Here's how the part is built. I have some questions about the finished solid (model axes, mm). A direction names the side the tool comes from. Round coordinates to 2 decimals unless told otherwise and drop trailing zeros. Order: outer loops, then holes, each group sorted by start corner. A loop starts at its lowest first (then second) coordinate and runs counter-clockwise, first axis right, second up. Notation, with made-up numbers: (-20, -25.5) - (-5, -25.5) arc R37 cw to (-5, 12.5) - close; hole circle Ø4 at (87, -37). An arc over 180 degrees is marked (long way). Answer as a JSON object with one key per item and string values.
```python
from build123d import *

# Parameters (mm, degrees)
CUT_EXTRUDE1_DEPTH = 27.095976701
CUT_EXTRUDE2_DEPTH = 3


with BuildPart() as part:
    # Sketch1 → Revolve2 (revolve)
    with BuildSketch(Plane.XY, mode=Mode.PRIVATE) as revolve2_sk:
        Polygon((0, 13), (15, 13), (15, 2), (16, 2), (16, 0), (0, 0), align=None)
    revolve(revolve2_sk.sketch.rotate(Axis((0, 0, 0), (0, 1, 0)), 90), axis=Axis((0, 0, 0), (0, 1, 0)))

    # Sketch2 → Cut-Extrude1 (cut, through all)
    with BuildSketch(Plane(origin=(0, 13, 0), x_dir=(1, 0, 0), z_dir=(0, 1, 0))):
        Polygon((-7, 0), (-3.5, -6.062177826), (3.5, -6.062177826), (7, 0), (3.5, 6.062177826), (-3.5, 6.062177826), align=None)
    extrude(amount=-CUT_EXTRUDE1_DEPTH, mode=Mode.SUBTRACT)

    # Sketch4 → Cut-Extrude2 (cut)
    with BuildSketch(Plane.XY.offset(15)):
        with BuildLine():
            Line((3, 9.5), (3, 5.5))
            ThreePointArc((3, 5.5), (0, 2.5), (-3, 5.5))
            Line((-3, 5.5), (-3, 9.5))
            ThreePointArc((-3, 9.5), (0, 12.5), (3, 9.5))
        make_face()
    extrude(amount=-CUT_EXTRUDE2_DEPTH, mode=Mode.SUBTRACT)


solid = part.part
```
1. Imagine slicing it at B-B (y = 9). List the corners of the cut face in (x, z) for me, plus the area to 3 significant figures.
Responses:
{"outline": "(-3, 12) - (-3, 14.7) arc R15 ccw (long way) to (3, 14.7) - (3, 12) - close; hole (-7, 0) - (-3.5, -6.06) - (3.5, -6.06) - (7, 0) - (3.5, 6.06) - (-3.5, 6.06) - close", "area": "562 mm2"}
2. Imagine slicing it at D-D (z = 14). List the corners of the cut face in (x, y) for me.
Responses:
{"outline": "(-7.75, 0) - (7.75, 0) - (7.75, 2) - (5.39, 2) - (5.39, 13) - (-5.39, 13) - (-5.39, 2) - (-7.75, 2) - close; hole (-3, 5.5) arc R3 ccw to (3, 5.5) - (3, 9.5) arc R3 ccw to (-3, 9.5) - close"}
3. For faces 4 (the face through (3, 8, 13)), 5 (the face through (0, 7, -6.062)), 6 (the face through (0, 0, -7)), which set-ups out of +Z, -Z, +X, -X, +Y, -Y let a thin tool reach every point of the face, with its end or its side?
Responses:
{"face 4": "+Z", "face 5": "+Y, -Y", "face 6": "+Z, -Z, +X, -X, -Y"}
4. For P1, Ø2, axis at y = 8.5, z = 13, coming from the -X side; P2, Ø3.5, axis at x = 0, y = 8, coming from the -Z side; P3, Ø3, axis at y = 9, z = -0.5, coming from the +X side, each with a flat end and sliding along its axis, tell me the tip position at first contact or that it passes through.
Responses:
{"P1": "x = -9", "P2": "z = -15", "P3": "x = 15"}
5. If I drill on L1, parallel to X at y = 5.5, z = 4; L2, parallel to Z at x = 6, y = 11; L3, parallel to X at y = 11.75, z = 2, over which ranges is the centre line in solid material (lowest first)? Write a range as [from, to].
Responses:
{"L1": "[-14.46, -4.69], [4.69, 14.46]", "L2": "[-13.75, -1.73], [1.73, 13.75]", "L3": "[-14.87, -5.85], [5.85, 14.87]"}
6. Imagine slicing it at A-A (x = 0). List the corners of the cut face in (y, z) for me.
Responses:
{"outline": "(0, -16) - (2, -16) - (2, -15) - (13, -15) - (13, -6.06) - (0, -6.06) - close; (0, 6.06) - (13, 6.06) - (13, 15) - (12.5, 15) - (12.5, 12) - (2.5, 12) - (2.5, 15) - (2, 15) - (2, 16) - (0, 16) - close"}
7. Thinking about a two-plate mould opening in X: for faces 1 (the face through (-0.2, 13, 6.5)), 2 (the face through (5.226, 6.591, 3.074)), 3 (the face through (-4.506, 7.423, -14.307)), which applies, pulls with the +X half, pulls with the -X half, needs draft (parallel to the pull), parting line crosses it, or undercut?
Responses:
{"face 1": "needs draft", "face 2": "undercut", "face 3": "parting line crosses it"}
8. Imagine slicing it at C-C (z = -1). List the corners of the cut face in (x, y) for me, plus the area to 3 significant figures.
Responses:
{"outline": "(-15.97, 0) - (-6.42, 0) - (-6.42, 13) - (-14.97, 13) - (-14.97, 2) - (-15.97, 2) - close; (6.42, 0) - (15.97, 0) - (15.97, 2) - (14.97, 2) - (14.97, 13) - (6.42, 13) - close", "area": "226 mm2"}
